from build123d import *

# Parameters (mm, degrees)
BOSS_EXTRUDE1_DEPTH = 3
SKETCH2_R           = 4.5
CUT_EXTRUDE1_DEPTH  = 74.927329182


with BuildPart() as part:
    # Sketch1 → Boss-Extrude1 (new body)
    with BuildSketch(Plane(origin=(0, 0, 0), x_dir=(0, 0, -1), z_dir=(1, 0, 0))):
        Polygon((0, 64.5), (-8.5, 64.5), (-8.5, 67.5), (-18.5, 67.5), (-18.5, 64.5), (-27, 64.5), (-27, 7.5), (-30, 7.5), (-30, -2.5), (-27, -2.5), (-27, -64.5), (-18.5, -64.5), (-18.5, -67.5), (-8.5, -67.5), (-8.5, -64.5), (0, -64.5), align=None)
    extrude(amount=BOSS_EXTRUDE1_DEPTH)

    # Sketch2 → Cut-Extrude1 (cut, through all)
    with BuildSketch(Plane(origin=(3, 0, 0), x_dir=(0, 0, -1), z_dir=(1, 0, 0))):
        with Locations((-15, 52.5)):
            Circle(SKETCH2_R)
        with Locations((-15, -52.5)):
            Circle(SKETCH2_R)
    extrude(amount=-CUT_EXTRUDE1_DEPTH, mode=Mode.SUBTRACT)


solid = part.part
Here's how the part is built. I have some questions about the finished solid (model axes, mm). A direction names the side the tool comes from. Round coordinates to 2 decimals unless told otherwise and drop trailing zeros. Order: outer loops, then holes, each group sorted by start corner. A loop starts at its lowest first (then second) coordinate and runs counter-clockwise, first axis right, second up. Notation, with made-up numbers: M 26,81 L 46,81 A19 cw 46,112 Z; hole C 50,-17 d11. An arc over 180 degrees is marked long. One line per question, with ' | ' between items.
1) On a 3-axis mill with a long thin cutter (end or side, diameter ignored), from which of +Z, -Z, +X, -X, +Y, -Y can I reach the whole of each face in a straight line? I mean faces 5 (the flat face through (1, 66, 8.5)), 6 (the flat face through (1, -64.5, 23)), 7 (the flat face through (1, -66, 8.5)), 8 (the flat face through (1, 7.5, 28)). Say none if no direction works.
Checked values:
face 5: -Z, +X, -X, +Y | face 6: +Z, +X, -X, -Y | face 7: -Z, +X, -X, -Y | face 8: +Z, +X, -X, +Y
2) We'd pull the mould along Y, two halves only. Please class faces 1 (the flat face through (1, 64.5, 23)), 2 (the cylindrical face through (1.52, -56.89, 15.98)), 3 (the flat face through (1, -33, 27)), 4 (the flat face through (1, -64.5, 4)): released by +Y, released by -Y, zero draft, split by the parting line, or undercut.
Checked values:
face 1: released by +Y | face 2: undercut | face 3: zero draft | face 4: released by -Y
3) I need wall thicknesses on line 1 (Y direction, x = 1.9, z = 15); line 2 (Y direction, x = 1.6, z = 26); line 3 (Y direction, x = 2.25, z = 12.25). Which ranges of each line are inside material? Lowest first, please.
Checked values:
line 1: y = -67.5 to -57, -48 to 48, 57 to 67.5 | line 2: y = -64.5 to 64.5 | line 3: y = -67.5 to -56.06, -48.94 to 48.94, 56.06 to 67.5
4) I'm going to push flat-ended pins straight in: pin 1 Ø1.5 at (x, y) = (1.5, -39) entering from +Z; pin 2 Ø1.5 at (x, z) = (1, 3.5) entering from -Y; pin 3 Ø0.9 at (x, z) = (2, 28) entering from +Y. Where does each tip first touch, or does it pass through?
Checked values:
pin 1: stops at z = 27 | pin 2: stops at y = -64.5 | pin 3: stops at y = 7.5
5) Imagine slicing it at C-C, the plane x = 2.2. Write out the boundary of the cut face in (y, z).
Checked values:
outline: M -67.5,8.5 L -64.5,8.5 L -64.5,0 L 64.5,0 L 64.5,8.5 L 67.5,8.5 L 67.5,18.5 L 64.5,18.5 L 64.5,27 L 7.5,27 L 7.5,30 L -2.5,30 L -2.5,27 L -64.5,27 L -64.5,18.5 L -67.5,18.5 Z; hole C -52.5,15 d9; hole C 52.5,15 d9
6) Imagine slicing it at D-D, the plane y = 12.5. Write out the boundary of the cut face in (x, z), plus the area to 3 significant figures.
Checked values:
outline: M 0,0 L 3,0 L 3,27 L 0,27 Z | area: 81.0 mm²
7) Imagine slicing it at B-B, the plane z = 15. Write out the boundary of the cut face in (x, y), plus the area to 3 significant figures.
Checked values:
outline: M 0,-67.5 L 3,-67.5 L 3,-57 L 0,-57 Z; M 0,-48 L 3,-48 L 3,48 L 0,48 Z; M 0,57 L 3,57 L 3,67.5 L 0,67.5 Z | area: 351 mm²
8) Imagine slicing it at A-A, the plane y = -52.5. Write out the boundary of the cut face in (x, z).
Checked values:
outline: M 0,0 L 3,0 L 3,10.5 L 0,10.5 Z; M 0,19.5 L 3,19.5 L 3,27 L 0,27 Z
